CAD build for the part. Positions are in the model's coordinates, mm. A direction names the side the tool comes from. Coordinates: 2 decimals unless noted, no trailing zeros. Loops run counter-clockwise (first coordinate to the right, second up) from the corner with the lowest first, then second, coordinate; pieces in that order, holes last. Notation, with made-up numbers: (66, -2.75) -> (123, -2.75) arc R15 ccw to (123, 23.25) -> close; hole circle Ø6 at (51.25, 52). An arc over 180 degrees is marked (long way). Answer as CSV lines item,"result". Start each with the question number.
from build123d import *

# Parameters (mm, degrees)
F1_START = -0.508
F0_R     = 11.90625
F0_R_2   = 4.92125
F1_DEPTH = 5.842
F0_R_3   = 1.19126
F2_DEPTH = 9.525
F3_SIZE  = 0.254


with BuildPart() as f1:
    # F0 (on Front) → F1 (new body)
    with BuildSketch(Plane.XZ.offset(F1_START)):
        Circle(F0_R)
        Circle(F0_R_2, mode=Mode.SUBTRACT)
    extrude(amount=-F1_DEPTH)

    # F0 (on Front) → F2 (join)
    with BuildSketch(Plane.XZ):
        Circle(F0_R_2)
        Circle(F0_R_3, mode=Mode.SUBTRACT)
    extrude(amount=-F2_DEPTH)

    # F3
    f3_edges = [f1.edges().sort_by_distance(p)[0] for p in [
        (-11.90625, 6.35, 0),
        (-11.90625, 0.508, 0),
        (-4.92125, 9.525, 0),
        (-4.92125, 6.35, 0),
    ]]
    chamfer(f3_edges, length=F3_SIZE)

    # F4 (on Right) → F5 (revolve, cut)
    with BuildSketch(Plane.YZ):
        Polygon((6.5216665858, 5.5874292748), (8.0233332929, 3.7639748771), (9.525, 5.5874292748), align=None)
    revolve(axis=Axis((0, 0, 0), (0, -1, 0)), mode=Mode.SUBTRACT)


solid = f1.part
Item 1: Saw through at C-C (y = 5.75). Write the cut outline in (x, z), plus the area to 3 significant figures.
Item 2: Flat gauge pins, fed straight in: pin 1 Ø2 at (x, z) = (-4, -5) entering from +Y; pin 2 Ø3 at (y, z) = (7, -7) entering from -X; pin 3 Ø4 at (x, y) = (-8, 6.5) entering from +Z. Where does each tip first touch, or does it go through?
Item 3: Which spindle directions (+Z, -Z, +X, -X, +Y, -Y) get a long thin tool onto all of the face, cutting with end or side? Do faces 1 (the face through (5, 6.35, -2)), 2 (the face through (1, 0, -1)), 3 (the face through (-3.9, 0.3, -3)). Say none if no direction does.
Item 4: Wall check: probe 1 along Z at (x, y) = (0, 4.75); probe 2 along Y at (x, z) = (5.75, -2.5); probe 3 along Y at (x, z) = (-1.25, -4) (3 decimals). Give the ranges that are in metal, low to high.
Geometry check:
1,outline,"circle Ø23.81 at (0, 0); hole circle Ø2.38 at (0, 0)"
1,area,"441 mm2"
2,pin 1,"y = 6.35"
2,pin 2,"x = -10.4"
2,pin 3,"z = 10.26"
3,face 1,"+Y"
3,face 2,"+Z, -Z, +X, -X, -Y"
3,face 3,"-Y"
4,probe 1,"-11.91 to -1.19, 1.19 to 11.91"
4,probe 2,"0.51 to 6.35"
4,probe 3,"0 to 7.672, 8.375 to 9.525"
